Print and shaded views of the part. All mm, measured from the part's lowest x, y and z. Round coordinates to 2 decimals unless told otherwise and drop trailing zeros. Loops run counter-clockwise (first coordinate to the right, second up) from the corner with the lowest first, then second, coordinate; pieces in that order, holes last. Notation, with made-up numbers: (-32, 14) -> (-7, 14) arc R3 cw to (-7, 18) -> close; hole circle Ø5 at (84, 56). An arc over 180 degrees is marked (long way). Use a Markdown table: item, result.
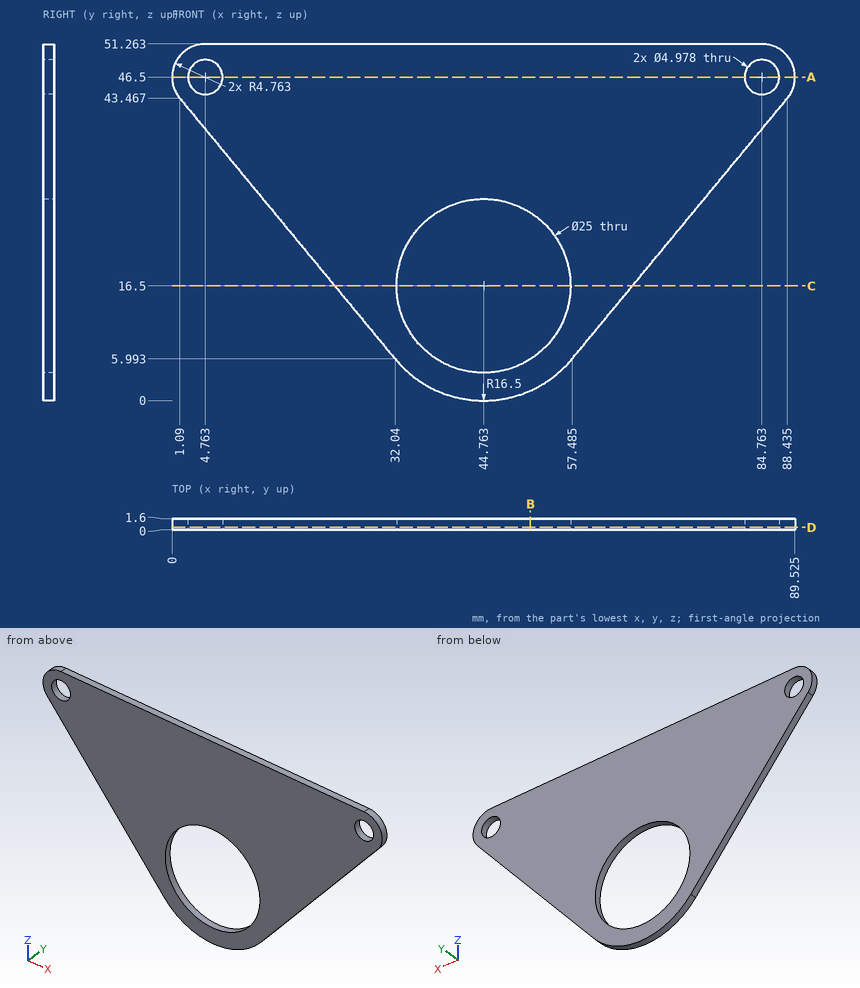
Q1. Band-saw the part on D-D, the plane y = 0.35. Give the cut face in (x, z) (1 decimal), plus the area to 3 significant figures.
Results list:
| item | result |
|---|---|
| outline | (1.1, 43.5) -> (32, 6) arc R16.5 ccw to (57.5, 6) -> (88.4, 43.5) arc R4.8 ccw to (84.8, 51.3) -> (4.8, 51.3) arc R4.8 ccw to start; hole circle Ø5 at (4.8, 46.5); hole circle Ø25 at (44.8, 16.5); hole circle Ø5 at (84.8, 46.5) |
| area | 2,380 mm² |
Q2. Drill centre lines: L1, parallel to X at y = 0.75, z = 46.5 (1 decimal); L2, parallel to Z at x = 44.5, y = 0.25; L3, parallel to Z at x = 41, y = 1.2 (1 decimal). Where is each one in solid material? Low to high. Write a range as from..to.
Results list:
| item | result |
|---|---|
| L1 | x = 0..2.3, 7.3..82.3, 87.3..89.5 |
| L2 | z = 0..4, 29..51.26 |
| L3 | z = 0.4..4.6, 28.4..51.3 |
Q3. Band-saw the part on C-C, the plane z = 16.5. Give the cut face in (x, y).
Results list:
| item | result |
|---|---|
| outline | (23.36, 0) -> (32.26, 0) -> (32.26, 1.6) -> (23.36, 1.6) -> close; (57.26, 0) -> (66.16, 0) -> (66.16, 1.6) -> (57.26, 1.6) -> close |
Q4. Band-saw the part on B-B, the plane x = 51.5. Give the cut face in (y, z).
Results list:
| item | result |
|---|---|
| outline | (0, 1.44) -> (1.6, 1.44) -> (1.6, 5.97) -> (0, 5.97) -> close; (0, 27.03) -> (1.6, 27.03) -> (1.6, 51.26) -> (0, 51.26) -> close |
Q5. Band-saw the part on A-A, the plane z = 46.5. Give the cut face in (x, y) (1 decimal).
Results list:
| item | result |
|---|---|
| outline | (0, 0) -> (2.3, 0) -> (2.3, 1.6) -> (0, 1.6) -> close; (7.3, 0) -> (82.3, 0) -> (82.3, 1.6) -> (7.3, 1.6) -> close; (87.3, 0) -> (89.5, 0) -> (89.5, 1.6) -> (87.3, 1.6) -> close |
Q6. Flat gauge pin, fed straight in: pin 1 (1.5 mm diameter, centred on x = 69, z = 25.5, fed in from -Y). Where does the tip first touch, or does it go through?
Results list:
| item | result |
|---|---|
| pin 1 | stops at y = 0 |
